Verification items for the finished model (mm, model axes). Face numbers are marked on the shaded views. A direction names the side the tool comes from. Coordinates: 2 decimals unless noted, no trailing zeros. Loops run counter-clockwise (first coordinate to the right, second up) from the corner with the lowest first, then second, coordinate; pieces in that order, holes last. Notation, with made-up numbers: (-15.5, 46) - (-8.5, 46) arc R9 cw to (-8.5, 51) - close; hole circle Ø10 at (5, 48.25). An arc over 180 degrees is marked (long way). One line per item, written item: value. Start each with the question number.
(1) Set-up check for the marked faces 5, 6, 7 and 8: record each of +Z, -Z, +X, -X, +Y, -Y from which the full face is reachable in a straight line by a thin tool's end or side.
(2) Gauge pin test, flat ends, axial feed: P1, Ø4, axis at x = -48, z = 39.5, coming from the +Y side; P2, Ø4, axis at x = -62, y = 25.5, coming from the +Z side; P3, Ø1.5, axis at x = -63.5, y = 23, coming from the -Z side. Record the tip position at first contact, or that the pin passes through.
(3) Section check B-B (y = 32). Record the boundary of the cut face in (x, z).
(4) Thickness scan on probe 1 along X at (y, z) = (16.5, 36.5); probe 2 along Z at (x, y) = (-37.85, 32); probe 3 along Y at (x, z) = (-44.25, 35.75). Record the ranges inside material, lowest first. Write a range as [from, to].
(5) Section check D-D (x = -44.5). Record the boundary of the cut face in (y, z), plus the area to 3 significant figures.
(6) Section check C-C (z = 44.25). Record the boundary of the cut face in (x, y), plus the area to 3 significant figures.
(7) Draft check along Y on the marked faces 1, 2, 3 and 4. Enter one of: +Y half, -Y half, draft (parallel to the pull), parting line (faces both ways), or undercut.
(8) Section check A-A (y = 11). Record the boundary of the cut face in (x, z).
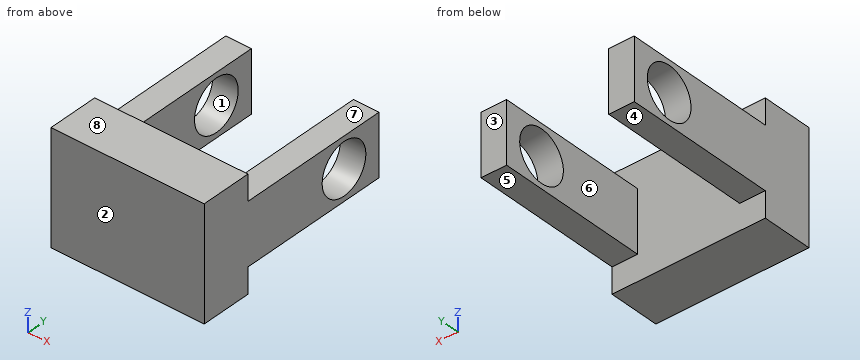
```python
from build123d import *

# Parameters (mm, degrees)
SKETCH1_W           = 30
SKETCH1_H           = 22
BOSS_EXTRUDE1_DEPTH = 10
SKETCH1_4_W         = 5
SKETCH1_4_H         = 12
BOSS_EXTRUDE2_DEPTH = 40
SKETCH2_R           = 5
CUT_EXTRUDE1_DEPTH  = 40


with BuildPart() as part:
    # Sketch1 → Boss-Extrude1 (new body)
    with BuildSketch(Plane(origin=(0, 0, 0), x_dir=(1, 0, 0), z_dir=(0, 1, 0))):
        with Locations((-50.637562945, -40.26337684)):
            Rectangle(SKETCH1_W, SKETCH1_H)
    extrude(amount=BOSS_EXTRUDE1_DEPTH)

    # Sketch1_4 → Boss-Extrude2 (add)
    with BuildSketch(Plane(origin=(0, 0, 0), x_dir=(1, 0, 0), z_dir=(0, 1, 0))):
        with Locations((-63.137562945, -40.26337684)):
            Rectangle(SKETCH1_4_W, SKETCH1_4_H)
        with Locations((-38.137562945, -40.26337684)):
            Rectangle(SKETCH1_4_W, SKETCH1_4_H)
    extrude(amount=BOSS_EXTRUDE2_DEPTH)

    # Sketch2 → Cut-Extrude1 (cut)
    with BuildSketch(Plane.ZY.offset(65.637562945)):
        with Locations(Location((40.26337684, 32, 0), (0, 0, 180))):
            Circle(SKETCH2_R)
    extrude(amount=-CUT_EXTRUDE1_DEPTH, mode=Mode.SUBTRACT)


solid = part.part
```
Responses:
1. face 5: -Z, +X, -X, +Y
1. face 6: +Z, -Z, +Y
1. face 7: +Z, +X, -X, +Y
1. face 8: +Z, +X, -X, +Y, -Y
2. P1: stops at y = 10
2. P2: stops at z = 46.26
2. P3: stops at z = 34.26
3. outline: (-65.64, 34.26) - (-60.64, 34.26) - (-60.64, 35.26) - (-65.64, 35.26) - close; (-65.64, 45.26) - (-60.64, 45.26) - (-60.64, 46.26) - (-65.64, 46.26) - close; (-40.64, 34.26) - (-35.64, 34.26) - (-35.64, 35.26) - (-40.64, 35.26) - close; (-40.64, 45.26) - (-35.64, 45.26) - (-35.64, 46.26) - (-40.64, 46.26) - close
4. probe 1: x = [-65.64, -60.64], [-40.64, -35.64]
4. probe 2: z = [34.26, 35.26], [45.26, 46.26]
4. probe 3: y = [0, 10]
5. outline: (0, 29.26) - (10, 29.26) - (10, 51.26) - (0, 51.26) - close
5. area: 220 mm²
6. outline: (-65.64, 0) - (-35.64, 0) - (-35.64, 28.98) - (-40.64, 28.98) - (-40.64, 10) - (-60.64, 10) - (-60.64, 28.98) - (-65.64, 28.98) - close; (-65.64, 35.02) - (-60.64, 35.02) - (-60.64, 40) - (-65.64, 40) - close; (-40.64, 35.02) - (-35.64, 35.02) - (-35.64, 40) - (-40.64, 40) - close
6. area: 540 mm²
7. face 1: undercut
7. face 2: -Y half
7. face 3: +Y half
7. face 4: draft
8. outline: (-65.64, 34.26) - (-60.64, 34.26) - (-60.64, 46.26) - (-65.64, 46.26) - close; (-40.64, 34.26) - (-35.64, 34.26) - (-35.64, 46.26) - (-40.64, 46.26) - close
